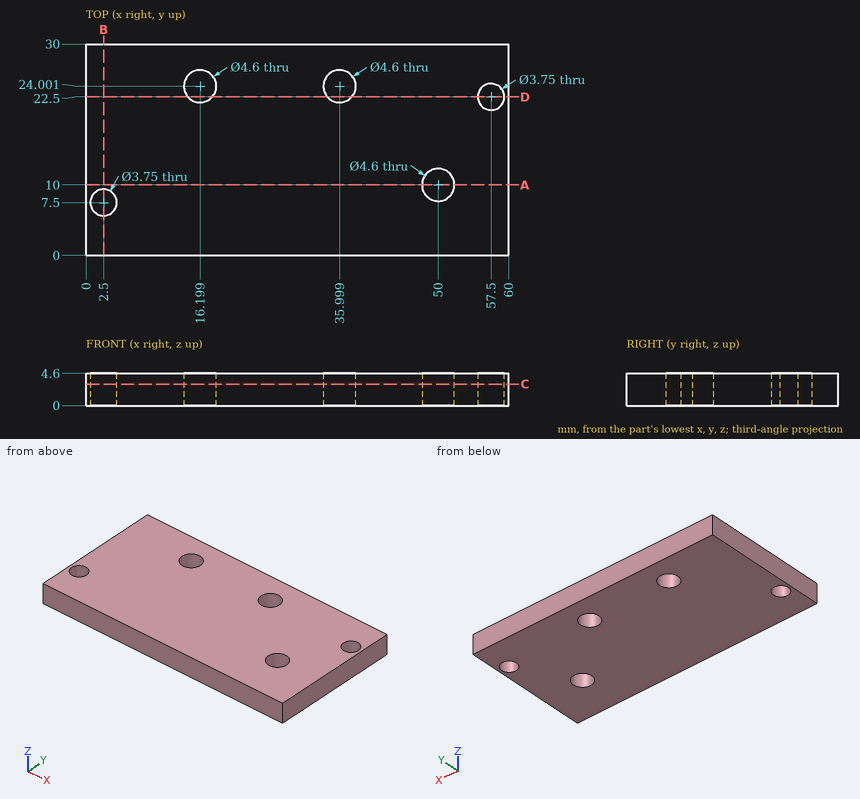
The drawing under review shows one solid part. Ordinate dimensions are in mm from its lowest x, y, z. Round coordinates to 2 decimals unless told otherwise and drop trailing zeros. Order: outer loops, then holes, each group sorted by start corner. A loop starts at its lowest first (then second) coordinate and runs counter-clockwise, first axis right, second up. Notation, with made-up numbers: (54, 21.5) -> (108, 21.5) arc R24 ccw to (108, 36.5) -> close; hole circle Ø7 at (25.25, -28). An arc over 180 degrees is marked (long way). Use a Markdown table: item, result.
Item 1: Take a section at C-C (z = 3.05). State how many separate pieces and enclosed holes the cut face has, plus the area to 3 significant figures.
Resolved:
| item | result |
|---|---|
| separate pieces | 1 |
| enclosed holes | 5 |
| area | 1,730 mm² |
Item 2: Take a section at A-A (y = 10). State the section outline as (x, z) points.
Resolved:
| item | result |
|---|---|
| outline | (0, 0) -> (47.7, 0) -> (47.7, 4.6) -> (0, 4.6) -> close; (52.3, 0) -> (60, 0) -> (60, 4.6) -> (52.3, 4.6) -> close |
Item 3: For line 1 along Y through (x, z) = (50, 1.45); line 2 along Y through (x, z) = (2.5, 1.5) (1 decimal); line 3 along X through (y, z) = (21.5, 2.9) (1 decimal), list the stretches that pass through material, from the lowest coordinate up. Write a range as [from, to].
Resolved:
| item | result |
|---|---|
| line 1 | y = [0, 7.7], [12.3, 30] |
| line 2 | y = [0, 5.6], [9.4, 30] |
| line 3 | x = [0, 55.9], [59.1, 60] |
Item 4: Take a section at D-D (y = 22.5). State the section outline as (x, z) points (1 decimal).
Resolved:
| item | result |
|---|---|
| outline | (0, 0) -> (14.5, 0) -> (14.5, 4.6) -> (0, 4.6) -> close; (17.9, 0) -> (34.3, 0) -> (34.3, 4.6) -> (17.9, 4.6) -> close; (37.7, 0) -> (55.6, 0) -> (55.6, 4.6) -> (37.7, 4.6) -> close; (59.4, 0) -> (60, 0) -> (60, 4.6) -> (59.4, 4.6) -> close |
Item 5: Take a section at B-B (x = 2.5). State the section outline as (y, z) points (1 decimal), plus the area to 3 significant figures.
Resolved:
| item | result |
|---|---|
| outline | (0, 0) -> (5.6, 0) -> (5.6, 4.6) -> (0, 4.6) -> close; (9.4, 0) -> (30, 0) -> (30, 4.6) -> (9.4, 4.6) -> close |
| area | 121 mm² |
